Read the model definition and answer for the solid it produces. Units are mm, in the model's axes. A direction names the side the tool comes from. Round coordinates to 2 decimals unless told otherwise and drop trailing zeros. Write each loop counter-clockwise with the first axis right and the second up, starting at its lowest first coordinate (ties: lowest second). Pieces come first, ordered by that corner, then holes. Notation, with made-up numbers: (74.25, 63) -> (78.25, 63) arc R27 cw to (78.25, 99) -> close; hole circle Ø4 at (-40, -33). An arc over 180 degrees is marked (long way). Return JSON: item names as keys, results as strings. Group by question number.
(1) A cutting plane is placed at C-C on z = -28. Give the vertices of the cut face in (x, y).
(2) A cutting plane is placed at B-B on x = 2.5. Give the vertices of the cut face in (y, z).
(3) Straight lines are drawn through the part: line 1 (Z direction, x = 5.75, y = -21); line 2 (Y direction, x = 2, z = -3). For each, find the intervals that lie inside material, in ascending order.
(4) The mould has two halves that part along Z. Classify faces 1 (the flat face through (4, -7, 42.25)), 2 (the flat face through (4, 7.594, -4)), 3 (the flat face through (4, -82.406, 5)): released by +Z, released by -Z, zero draft, split by the parting line, or undercut.
(5) A cutting plane is placed at A-A on y = -34.5. Give the vertices of the cut face in (x, z), then the cut area to 3 significant figures.
(6) For faces 4 (the flat face through (4, -18, -8.75)), 5 (the flat face through (0, -21, 1)), 6 (the flat face through (4, -52.406, -31)), determine the directions among +Z, -Z, +X, -X, +Y, -Y from which every point of the face is accessible in a straight line to the end or side of a thin tool.
(7) A cutting plane is placed at D-D on y = -63. Give the vertices of the cut face in (x, z), then the cut area to 3 significant figures.
(8) Given pin 1 (7.5 mm diameter, centred on y = 17.59, z = 30.25, fed in from -X); pin 2 (2.5 mm diameter, centred on x = 6, z = -26, fed in from -Y); pin 3 (4 mm diameter, centred on x = 1.5, z = 29.5, fed in from -Y), each flat-ended and moving along its own axis, determine where each tip first touches the part or whether it passes through.
```python
from build123d import *

# Parameters (mm, degrees)
F0_W     = 50
F0_H     = 8.75
F1_DEPTH = 8


with BuildPart() as f1:
    # F0 (on Right) → F1 (new body)
    with BuildSketch(Plane.YZ):
        with BuildLine():
            Line((17.593615, 42.25), (-19.906385, 42.25))
            Line((-19.906385, 42.25), (-57.406385, 42.25))
            ThreePointArc((-57.406385, 42.25), (-75.084055, 34.92767), (-82.406385, 17.25))
            Line((-82.406385, 17.25), (-82.406385, -7.25))
            ThreePointArc((-82.406385, -7.25), (-79.504872, -14.254872), (-72.5, -17.156385))
            Line((-72.5, -17.156385), (-52.406385, -17.156385))
            Line((-52.406385, -17.156385), (-44.993822, -10.444165))
            ThreePointArc((-44.993822, -10.444165), (-43.180784, -10.581559), (-43.412569, -12.384961))
            Line((-43.412569, -12.384961), (-50.909492, -19.173572))
            Line((-50.909492, -19.173572), (-52.406385, -20.379891))
            Line((-52.406385, -20.379891), (-52.406385, -42.25))
            Line((-52.406385, -42.25), (42.593615, -42.25))
            Line((42.593615, -42.25), (42.593615, 0))
            Line((42.593615, 0), (42.593615, 42.25))
            Line((42.593615, 42.25), (17.593615, 42.25))
        make_face()
        with Locations((-17.406385, -4.375)):
            Rectangle(F0_W, F0_H, mode=Mode.SUBTRACT)
        with BuildLine():
            ThreePointArc((20.923833, 30.25), (15.238794, 27.89518), (17.593615, 33.580219))
            ThreePointArc((17.593615, 33.580219), (19.948435, 32.60482), (20.923833, 30.25))
        make_face(mode=Mode.SUBTRACT)
    extrude(amount=F1_DEPTH)


solid = f1.part
```
Checks:
{
 "1": {"outline": "(0, -52.41) -> (8, -52.41) -> (8, 42.59) -> (0, 42.59) -> close"},
 "2": {"outline": "(-82.41, -7.25) arc R9.91 ccw to (-72.5, -17.16) -> (-52.41, -17.16) -> (-44.99, -10.44) arc R1.25 cw (long way) to (-43.41, -12.38) -> (-50.91, -19.17) -> (-52.41, -20.38) -> (-52.41, -42.25) -> (42.59, -42.25) -> (42.59, 42.25) -> (-57.41, 42.25) arc R25 ccw to (-82.41, 17.25) -> close; hole (-42.41, -8.75) -> (7.59, -8.75) -> (7.59, 0) -> (-42.41, 0) -> close; hole circle Ø6.66 at (17.59, 30.25)"},
 "3": {"line 1": "z = -42.25 to -8.75, 0 to 42.25", "line 2": "y = -82.41 to -42.41, 7.59 to 42.59"},
 "4": {"face 1": "released by +Z", "face 2": "undercut", "face 3": "zero draft"},
 "5": {"outline": "(0, -42.25) -> (8, -42.25) -> (8, -8.75) -> (0, -8.75) -> close; (0, 0) -> (8, 0) -> (8, 42.25) -> (0, 42.25) -> close", "area": "606 mm^2"},
 "6": {"face 4": "+X, -X", "face 5": "+Z, -Z, -X, +Y, -Y", "face 6": "-Z, +X, -X, -Y"},
 "7": {"outline": "(0, -17.16) -> (8, -17.16) -> (8, 41.62) -> (0, 41.62) -> close", "area": "470 mm^2"},
 "8": {"pin 1": "stops at x = 0", "pin 2": "stops at y = -52.41", "pin 3": "stops at y = -80.21"}
}
